Check sheet for the drawn part. Datum: minimum x, y, z corner. Units: mm. A direction names the side the tool comes from. Coordinates: 2 decimals unless noted, no trailing zeros. Loops run counter-clockwise (first coordinate to the right, second up) from the corner with the lowest first, then second, coordinate; pieces in that order, holes last. Notation, with made-up numbers: M 60.5,48.5 L 68.5,48.5 A32 ccw 68.5,87.5 Z; hole C -9.5,8 d9. An arc over 180 degrees is marked long. Answer in a Markdown table with one row per item. Add a question column.
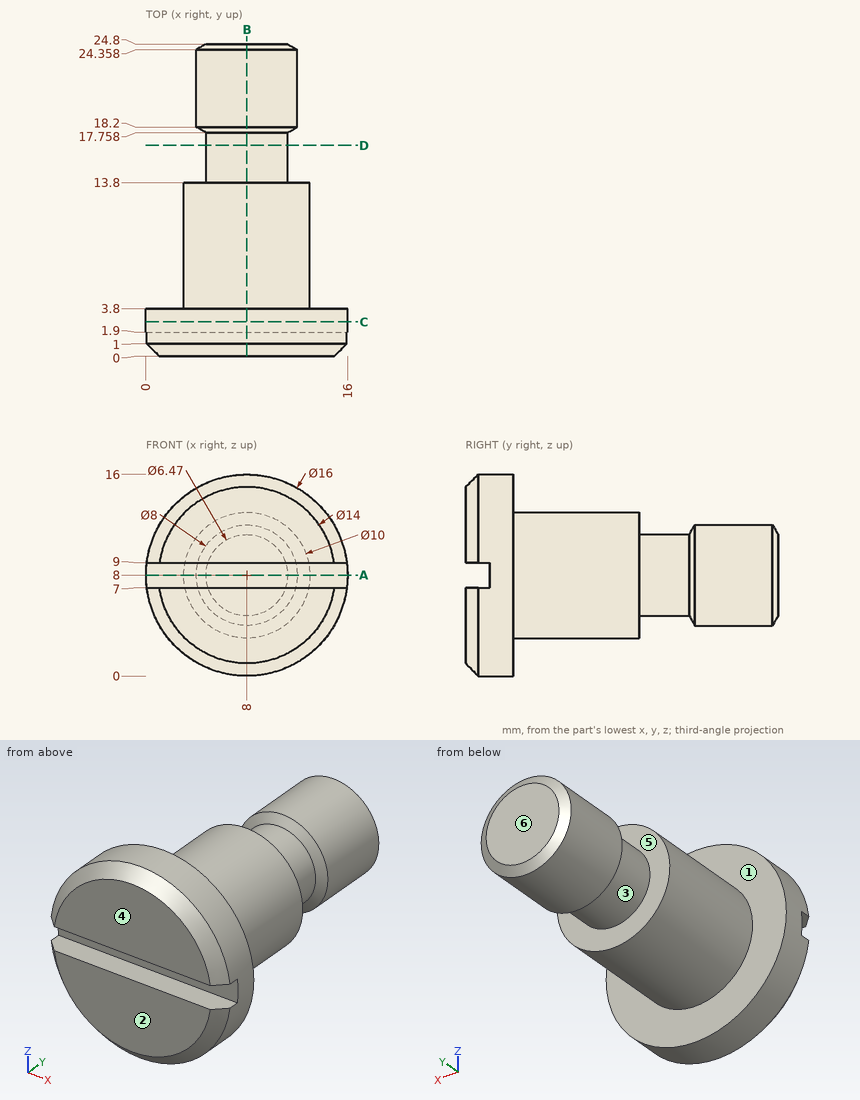
Q1. Thickness scan on L1, parallel to Y at x = 13, z = 10.5; L2, parallel to Y at x = 15.25, z = 8; L3, parallel to X at y = 7.75, z = 7. Record the ranges inside material, lowest first.
Q2. Access from +Z, -Z, +X, -X, +Y, -Y to the whole of each face (thin tool, end or side, straight path). Record for the marked faces 1, 2 and 3.
Q3. Go/stop test with flat-tipped pins: pin 1 (8 mm diameter, centred on y = 18, z = 5, fed in from +X); pin 2 (0.6 mm diameter, centred on x = 5, y = 1.5, fed in from +Z); pin 3 (1.5 mm diameter, centred on x = 13.5, y = 20, fed in from -Z); pin 4 (0.6 mm diameter, centred on x = 10, z = 8.5, fed in from -Y). Record where each tip stops, or that it passes through.
Q4. Mould release check, pull along Y, two halves, no side actions. Record for the marked faces 4, 5 and 6: released by +Y, released by -Y, zero draft, split by the parting line, or undercut.
Q5. Cross-section at A-A (z = 8). Record the cut outline in (x, y) (1 decimal).
Q6. Cross-section at D-D (y = 16.75). Record the cut outline in (x, z) (1 decimal), plus the area to 3 significant figures.
Q7. Cross-section at C-C (y = 2.75). Record the cut outline in (x, z).
Q8. Cross-section at B-B (x = 8). Record the cut outline in (y, z) (1 decimal).
Answer key:
| question | item | result |
|---|---|---|
| 1 | L1 | 0 to 3.8 |
| 1 | L2 | 1.9 to 3.8 |
| 1 | L3 | 3.1 to 12.9 |
| 2 | face 1 | +Y |
| 2 | face 2 | +Z, -Z, +X, -X, -Y |
| 2 | face 3 | none |
| 3 | pin 1 | x = 12 |
| 3 | pin 2 | z = 15.53 |
| 3 | pin 3 | through |
| 3 | pin 4 | y = 1.9 |
| 4 | face 4 | released by -Y |
| 4 | face 5 | undercut |
| 4 | face 6 | released by +Y |
| 5 | outline | M 0,1.9 L 16,1.9 L 16,3.8 L 13,3.8 L 13,13.8 L 11.2,13.8 L 11.2,17.8 L 12,18.2 L 12,24.4 L 11.2,24.8 L 4.8,24.8 L 4,24.4 L 4,18.2 L 4.8,17.8 L 4.8,13.8 L 3,13.8 L 3,3.8 L 0,3.8 Z |
| 6 | outline | C 8,8 d6.5 |
| 6 | area | 32.9 mm^2 |
| 7 | outline | C 8,8 d16 |
| 8 | outline | M 0,1 L 1,0 L 3.8,0 L 3.8,3 L 13.8,3 L 13.8,4.8 L 17.8,4.8 L 18.2,4 L 24.4,4 L 24.8,4.8 L 24.8,11.2 L 24.4,12 L 18.2,12 L 17.8,11.2 L 13.8,11.2 L 13.8,13 L 3.8,13 L 3.8,16 L 1,16 L 0,15 L 0,9 L 1.9,9 L 1.9,7 L 0,7 Z |
